Work out the finished part from the listing and answer in its coordinate system (mm). A direction names the side the tool comes from. Coordinates: 2 decimals unless noted, no trailing zeros. Write each question's results on one line, items separated by ' | '. Start each with the question number.
1. Find the intervals of material crossed by line 1 along X through (y, z) = (3.3, 0); line 2 along Z through (x, y) = (12, 4.35); line 3 along X through (y, z) = (1.9, 2), in increasing order. Write a range as [from, to].
2. Each of these flat-tipped pins is pushed along its axis until it touches: P1, Ø3, axis at x = -24.5, z = 1.5, coming from the +Y side; P2, Ø2, axis at y = 4, z = 13, coming from the -X side; P3, Ø2.5, axis at x = 78.5, y = 1.5, coming from the -Z side. Where does it stop, or does it pass through?
3. A cutting plane is placed at A-A on y = 1.65. State how many separate pieces and enclosed holes the cut face has, then the cut area to 3 significant figures.
4. Which of the six approach directions +Z, -Z, +X, -X, +Y, -Y give full straight-line access (tool end or side, diameter ignored) to faces 1 (the flat face through (63, 2, -27.774)), 2 (the flat face through (23.6, 3.5, 1.4))?
from build123d import *

# Parameters (mm, degrees)
BOSS_EXTRUDE3_OUTLINE_R   = 17.5
BOSS_EXTRUDE3_OUTLINE_R_2 = 7.6
BOSS_EXTRUDE3_DEPTH       = 5
SKETCH2_R                 = 1.6
CUT_EXTRUDE1_DEPTH        = 10
SKETCH3_R                 = 1.6
CUT_EXTRUDE2_DEPTH        = 10
SKETCH4_R                 = 1.6
CUT_EXTRUDE3_DEPTH        = 10
SKETCH5_R                 = 3.25
CUT_EXTRUDE5_DEPTH        = 1.5
CUT_EXTRUDE6_DEPTH        = 10
FILLET3_R                 = 2
FILL_PATTERN2_DEPTH       = 5
CUT_EXTRUDE7_DEPTH        = 10
FILLET4_R                 = 2
FILL_PATTERN4_DEPTH       = 5


# Read off the part's stored shape, not the designer's step: Boss-Extrude3, Fill Pattern2, Fill Pattern4
with BuildPart() as part:
    # Boss-Extrude3 outline → Boss-Extrude3 (new body)
    with BuildSketch(Plane(origin=(0, 0, 0), x_dir=(1, 0, 0), z_dir=(0, 1, 0))):
        with BuildLine():
            ThreePointArc((0, 42.5), (-42.5, 0), (0, -42.5))
            add(Edge.make_bspline(
                [(0, -42.5), (50, -42.5), (76.766110149, 8.415768242), (141.161165235, -8.838834765)],
                knots=[0, 0, 0, 0, 1, 1, 1, 1], degree=3))
            ThreePointArc((141.161165235, -8.838834765), (158.838834765, -8.838834765), (158.838834765, 8.838834765))
            add(Edge.make_bspline(
                [(0, 42.5), (53.483495706, 42.5), (123.483495706, 44.194173824), (158.838834765, 8.838834765)],
                knots=[0, 0, 0, 0, 1, 1, 1, 1], degree=3))
        make_face()
        Circle(BOSS_EXTRUDE3_OUTLINE_R, mode=Mode.SUBTRACT)
        with Locations((150, 0)):
            Circle(BOSS_EXTRUDE3_OUTLINE_R_2, mode=Mode.SUBTRACT)
    extrude(amount=BOSS_EXTRUDE3_DEPTH)

    # Sketch2 → Cut-Extrude1 (cut)
    with BuildSketch(Plane(origin=(0, 5, 0), x_dir=(1, 0, 0), z_dir=(0, 1, 0))):
        with Locations(Location((0, 35, 0), (0, 0, 270))):
            Circle(SKETCH2_R)
        with Locations(Location((0, 25, 0), (0, 0, 270))):
            Circle(SKETCH2_R)
        with Locations(Location((12.5, 21.650635095, 0), (0, 0, 270))):
            Circle(SKETCH2_R)
        with Locations(Location((21.650635095, 12.5, 0), (0, 0, 270))):
            Circle(SKETCH2_R)
        with Locations(Location((25, 0, 0), (0, 0, 270))):
            Circle(SKETCH2_R)
        with Locations(Location((21.650635095, -12.5, 0), (0, 0, 270))):
            Circle(SKETCH2_R)
        with Locations(Location((12.5, -21.650635095, 0), (0, 0, 270))):
            Circle(SKETCH2_R)
        with Locations(Location((0, -25, 0), (0, 0, 270))):
            Circle(SKETCH2_R)
        with Locations(Location((-12.5, -21.650635095, 0), (0, 0, 270))):
            Circle(SKETCH2_R)
        with Locations(Location((-21.650635095, -12.5, 0), (0, 0, 270))):
            Circle(SKETCH2_R)
        with Locations(Location((-25, 0, 0), (0, 0, 270))):
            Circle(SKETCH2_R)
        with Locations(Location((-21.650635095, 12.5, 0), (0, 0, 270))):
            Circle(SKETCH2_R)
        with Locations(Location((-12.5, 21.650635095, 0), (0, 0, 270))):
            Circle(SKETCH2_R)
        with Locations(Location((-20.57248383, 28.315594803, 0), (0, 0, 270))):
            Circle(SKETCH2_R)
        with Locations(Location((-33.28697807, 10.815594803, 0), (0, 0, 270))):
            Circle(SKETCH2_R)
        with Locations(Location((-33.28697807, -10.815594803, 0), (0, 0, 270))):
            Circle(SKETCH2_R)
        with Locations(Location((-20.57248383, -28.315594803, 0), (0, 0, 270))):
            Circle(SKETCH2_R)
        with Locations(Location((0, -35, 0), (0, 0, 270))):
            Circle(SKETCH2_R)
    extrude(amount=-CUT_EXTRUDE1_DEPTH, mode=Mode.SUBTRACT)

    # Sketch3 → Cut-Extrude2 (cut)
    with BuildSketch(Plane(origin=(0, 5, 0), x_dir=(1, 0, 0), z_dir=(0, 1, 0))):
        with Locations(Location((29.822508304, 35, 0), (0, 0, 270))):
            Circle(SKETCH3_R)
        with Locations(Location((57.312909887, 35, 0), (0, 0, 270))):
            Circle(SKETCH3_R)
    extrude(amount=-CUT_EXTRUDE2_DEPTH, mode=Mode.SUBTRACT)

    # Sketch4 → Cut-Extrude3 (cut)
    with BuildSketch(Plane(origin=(0, 5, 0), x_dir=(1, 0, 0), z_dir=(0, 1, 0))):
        with Locations(Location((22.392043347, -28.36049342, 0), (0, 0, 270))):
            Circle(SKETCH4_R)
    extrude(amount=-CUT_EXTRUDE3_DEPTH, mode=Mode.SUBTRACT)

    # Sketch5 → Cut-Extrude5 (cut)
    with BuildSketch(Plane(origin=(0, 5, 0), x_dir=(1, 0, 0), z_dir=(0, 1, 0))):
        with Locations(Location((25, 0, 0), (0, 0, 270))):
            Circle(SKETCH5_R)
        with Locations(Location((12.5, -21.650635095, 0), (0, 0, 270))):
            Circle(SKETCH5_R)
        with Locations(Location((-12.5, -21.650635095, 0), (0, 0, 270))):
            Circle(SKETCH5_R)
        with Locations(Location((-25, 0, 0), (0, 0, 270))):
            Circle(SKETCH5_R)
        with Locations(Location((-12.5, 21.650635095, 0), (0, 0, 270))):
            Circle(SKETCH5_R)
        with Locations(Location((12.5, 21.650635095, 0), (0, 0, 270))):
            Circle(SKETCH5_R)
    extrude(amount=-CUT_EXTRUDE5_DEPTH, mode=Mode.SUBTRACT)

    # Sketch6 → Cut-Extrude6 (cut)
    with BuildSketch(Plane(origin=(0, 5, 0), x_dir=(1, 0, 0), z_dir=(0, 1, 0))):
        Polygon((43, 27.773502692), (23, 27.773502692), (33, 10.452994616), align=None)
    extrude(amount=-CUT_EXTRUDE6_DEPTH, mode=Mode.SUBTRACT)

    # Fillet3
    fillet3_edges = [part.edges().sort_by_distance(p)[0] for p in [
        (43, 2.5, -27.773502692),
        (33, 2.5, -10.452994616),
        (23, 2.5, -27.773502692),
    ]]
    fillet(fillet3_edges, radius=FILLET3_R)

    # Fill Pattern2 outline → Fill Pattern2 (cut)
    with BuildSketch(Plane(origin=(0, 0, 0), x_dir=(1, 0, 0), z_dir=(0, 1, 0))):
        with BuildLine():
            ThreePointArc((41.464101615, 1.792740578), (39.732050808, 0.792740578), (39.732050808, -1.207259422))
            Line((39.732050808, -1.207259422), (46.267949192, -12.527767497))
            ThreePointArc((46.267949192, -12.527767497), (48, -13.527767497), (49.732050808, -12.527767497))
            Line((49.732050808, -12.527767497), (56.267949192, -1.207259422))
            ThreePointArc((56.267949192, -1.207259422), (56.267949192, 0.792740578), (54.535898385, 1.792740578))
            Line((54.535898385, 1.792740578), (41.464101615, 1.792740578))
        make_face()
        with BuildLine():
            ThreePointArc((101.267949192, 24.773502692), (101.267949192, 26.773502692), (99.535898385, 27.773502692))
            Line((99.535898385, 27.773502692), (86.464101615, 27.773502692))
            ThreePointArc((86.464101615, 27.773502692), (84.732050808, 26.773502692), (84.732050808, 24.773502692))
            Line((84.732050808, 24.773502692), (91.267949192, 13.452994616))
            ThreePointArc((91.267949192, 13.452994616), (93, 12.452994616), (94.732050808, 13.452994616))
            Line((94.732050808, 13.452994616), (101.267949192, 24.773502692))
        make_face()
        with BuildLine():
            ThreePointArc((71.267949192, 24.773502692), (71.267949192, 26.773502692), (69.535898385, 27.773502692))
            Line((69.535898385, 27.773502692), (56.464101615, 27.773502692))
            ThreePointArc((56.464101615, 27.773502692), (54.732050808, 26.773502692), (54.732050808, 24.773502692))
            Line((54.732050808, 24.773502692), (61.267949192, 13.452994616))
            ThreePointArc((61.267949192, 13.452994616), (63, 12.452994616), (64.732050808, 13.452994616))
            Line((64.732050808, 13.452994616), (71.267949192, 24.773502692))
        make_face()
    extrude(amount=FILL_PATTERN2_DEPTH, mode=Mode.SUBTRACT)

    # Sketch7 → Cut-Extrude7 (cut)
    with BuildSketch(Plane(origin=(0, 5, 0), x_dir=(1, 0, 0), z_dir=(0, 1, 0))):
        Polygon((58, 7.56624327), (48, 24.886751346), (38, 7.56624327), align=None)
    extrude(amount=-CUT_EXTRUDE7_DEPTH, mode=Mode.SUBTRACT)

    # Fillet4
    fillet4_edges = [part.edges().sort_by_distance(p)[0] for p in [
        (58, 2.5, -7.56624327),
        (38, 2.5, -7.56624327),
        (48, 2.5, -24.886751346),
    ]]
    fillet(fillet4_edges, radius=FILLET4_R)

    # Fill Pattern4 outline → Fill Pattern4 (cut)
    with BuildSketch(Plane(origin=(0, 0, 0), x_dir=(1, 0, 0), z_dir=(0, 1, 0))):
        with BuildLine():
            ThreePointArc((69.732050808, 10.56624327), (69.732050808, 8.56624327), (71.464101615, 7.56624327))
            Line((71.464101615, 7.56624327), (84.535898385, 7.56624327))
            ThreePointArc((84.535898385, 7.56624327), (86.267949192, 8.56624327), (86.267949192, 10.56624327))
            Line((86.267949192, 10.56624327), (79.732050808, 21.886751346))
            ThreePointArc((79.732050808, 21.886751346), (78, 22.886751346), (76.267949192, 21.886751346))
            Line((76.267949192, 21.886751346), (69.732050808, 10.56624327))
        make_face()
    extrude(amount=FILL_PATTERN4_DEPTH, mode=Mode.SUBTRACT)


solid = part.part
Values:
1) line 1: [-42.5, -26.6], [-23.4, -17.5], [17.5, 23.4], [26.6, 39.47], [56.53, 142.4], [157.6, 162.5] | line 2: [-42.51, -24.86], [-18.44, -12.74], [12.74, 18.44], [24.86, 41.52] | line 3: [-42.45, -17.39], [17.39, 40.19], [55.81, 142.67], [157.33, 162.34]
2) P1: y = 3.5 | P2: x = -40.77 | P3: z = -40.03
3) separate pieces: 1 | enclosed holes: 29 | area: 9,320 mm^2
4) face 1: +Y, -Y | face 2: +Y
